```python
from build123d import *

# Parameters (mm, degrees)
SKETCH1_W             = 76.2
SKETCH1_H             = 50.8
BOSS_EXTRUDE1_DEPTH   = 27.94
SKETCH2_R             = 6.985
SKETCH2_R_2           = 9
CUT_EXTRUDE1_DEPTH    = 28.94
CUT_EXTRUDE2_DEPTH    = 21.59
M3_CLEARANCE_HOLE1_D  = 3.4
F_6_CLEARANCE_HOLE1_D = 3.7973


with BuildPart() as part:
    # Sketch1 → Boss-Extrude1 (new body)
    with BuildSketch(Plane(origin=(0, 0, 0), x_dir=(1, 0, 0), z_dir=(0, 1, 0))):
        Rectangle(SKETCH1_W, SKETCH1_H)
    extrude(amount=BOSS_EXTRUDE1_DEPTH)

    # Sketch2 → Cut-Extrude1 (cut, through all)
    with BuildSketch(Plane.XZ):
        with Locations((-9.525, 0)):
            Circle(SKETCH2_R)
        with Locations((9.525, 0)):
            Circle(SKETCH2_R_2)
    extrude(amount=-CUT_EXTRUDE1_DEPTH, mode=Mode.SUBTRACT)

    # Sketch3 → Cut-Extrude2 (cut)
    with BuildSketch(Plane(origin=(0, 27.94, 0), x_dir=(1, 0, 0), z_dir=(0, 1, 0))):
        with BuildLine():
            Line((-12.7, -19.05), (12.7, -19.05))
            ThreePointArc((12.7, -19.05), (21.680256121, -15.330256121), (25.4, -6.35))
            Line((25.4, -6.35), (25.4, 6.35))
            ThreePointArc((25.4, 6.35), (21.680256121, 15.330256121), (12.7, 19.05))
            Line((12.7, 19.05), (-12.7, 19.05))
            ThreePointArc((-12.7, 19.05), (-21.680256121, 15.330256121), (-25.4, 6.35))
            Line((-25.4, 6.35), (-25.4, -6.35))
            ThreePointArc((-25.4, -6.35), (-21.680256121, -15.330256121), (-12.7, -19.05))
        make_face()
    extrude(amount=-CUT_EXTRUDE2_DEPTH, mode=Mode.SUBTRACT)

    # M3 Clearance Hole1 (through all)
    with Locations(Plane(origin=(0.332611845, 0, 9.192388155), x_dir=(0, 0, -1), z_dir=(0, -1, 0))):
        with Locations((0, 0), (18.38477631, 0), (0, 18.38477631), (18.38477631, 18.38477631)):
            Hole(M3_CLEARANCE_HOLE1_D / 2)

    # #6 Clearance Hole1 (through all)
    with Locations(Plane(origin=(-31.75, 0, 15.875), x_dir=(0, 0, -1), z_dir=(0, -1, 0))):
        with Locations((0, 0), (31.75, 0), (0, 63.5), (31.75, 63.5)):
            Hole(F_6_CLEARANCE_HOLE1_D / 2)


solid = part.part
```
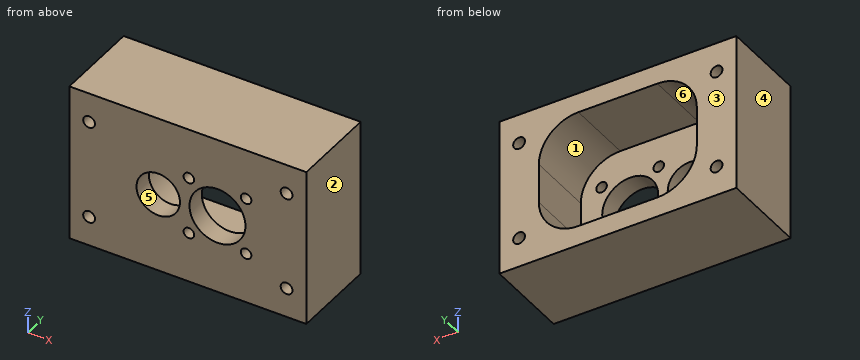
For this review, take the finished solid that the model builds, in its own axes (mm). Face numbers are marked on the shaded views. A direction names the side the tool comes from. Round coordinates to 2 decimals unless told otherwise and drop trailing zeros. Write each loop counter-clockwise with the first axis right and the second up, starting at its lowest first coordinate (ties: lowest second). Pieces come first, ordered by that corner, then holes. Notation, with made-up numbers: M 50,40.25 L 96,40.25 A20 ccw 96,65.25 Z; hole C 28.25,53 d4. An arc over 180 degrees is marked long. One line per item, written item: value. Start each with the question number.
(1) Machinability: for the marked faces 5 and 6, which of the approach directions +Z, -Z, +X, -X, +Y, -Y give a long, thin tool a straight path to every point of the face, cutting with its end or side? Answer none if there is none.
(2) Insertion check: pin 1 (18 mm diameter, centred on x = -9.525, z = 0, fed in from +Y); pin 2 (2.5 mm diameter, centred on x = 31.75, z = 15.875, fed in from -Y); pin 3 (12 mm diameter, centred on x = 11, z = 19, fed in from -Y). Each pin has a flat end and moves straight along its axis. Give the tip position at first contact, or say it passes through.
(3) We need section D-D (y = 19.25). Give the boundary of the cut face in (x, z) (3 decimals), and give its area (3 significant figures).
(4) We need section B-B (z = 0). Give the boundary of the cut face in (x, y) (3 decimals).
(5) Wall thickness on line 1 (Z direction, x = 32, y = 25.25); line 2 (Z direction, x = -11, y = 22.5); line 3 (X direction, y = 23, z = 3): over which ranges is each line inside the solid? List them lowest first.
(6) The part is to be moulded in two halves that separate along X. For the marked faces 1, 2, 3 and 4, say which applies: released by +X, released by -X, zero draft, split by the parting line, or undercut.
(7) We need section A-A (x = -31.75). Give the boundary of the cut face in (y, z), and give its area (3 significant figures).
(8) We need section C-C (x = 3). Give the boundary of the cut face in (y, z).
Result:
1. face 5: +Y, -Y
1. face 6: +Y
2. pin 1: y = 6.35
2. pin 2: through
2. pin 3: y = 0
3. outline: M -38.1,-25.4 L 38.1,-25.4 L 38.1,25.4 L -38.1,25.4 Z; hole C -31.75,-15.875 d3.797; hole C -31.75,15.875 d3.797; hole M -25.4,-6.35 A12.7 ccw -12.7,-19.05 L 12.7,-19.05 A12.7 ccw 25.4,-6.35 L 25.4,6.35 A12.7 ccw 12.7,19.05 L -12.7,19.05 A12.7 ccw -25.4,6.35 Z; hole C 31.75,-15.875 d3.797; hole C 31.75,15.875 d3.797
3. area: 2,030 mm²
4. outline: M -38.1,0 L -16.51,0 L -16.51,6.35 L -25.4,6.35 L -25.4,27.94 L -38.1,27.94 Z; M -2.54,0 L 0.525,0 L 0.525,6.35 L -2.54,6.35 Z; M 18.525,0 L 38.1,0 L 38.1,27.94 L 25.4,27.94 L 25.4,6.35 L 18.525,6.35 Z
5. line 1: -25.4 to -17.76, -13.99 to 13.99, 17.76 to 25.4
5. line 2: -25.4 to -19.05, 19.05 to 25.4
5. line 3: -38.1 to -25.4, 25.4 to 38.1
6. face 1: undercut
6. face 2: released by +X
6. face 3: zero draft
6. face 4: released by -X
7. outline: M 0,-25.4 L 27.94,-25.4 L 27.94,-17.77 L 0,-17.77 Z; M 0,-13.98 L 27.94,-13.98 L 27.94,13.98 L 0,13.98 Z; M 0,17.77 L 27.94,17.77 L 27.94,25.4 L 0,25.4 Z
7. area: 1,210 mm²
8. outline: M 0,-25.4 L 27.94,-25.4 L 27.94,-19.05 L 6.35,-19.05 L 6.35,-6.2 L 0,-6.2 Z; M 0,6.2 L 6.35,6.2 L 6.35,19.05 L 27.94,19.05 L 27.94,25.4 L 0,25.4 Z
